Could you check a few things on this model? Use its own coordinates, in mm. A direction names the side the tool comes from. Coordinates: 2 decimals unless noted, no trailing zeros. Order: outer loops, then holes, each group sorted by start corner. A loop starts at its lowest first (then second) coordinate and runs counter-clockwise, first axis right, second up.
```python
from build123d import *

# Parameters (mm, degrees)
F0_R     = 20.955
F1_DEPTH = 6.35
F3_R     = 13.97
F4_DEPTH = 38.1
F5_R     = 7.62
F2_R     = 1.905
F7_DEPTH = 2.54
F6_R     = 1.905
F8_DEPTH = 2.54


with BuildPart() as f1:
    # F0 (on Top) → F1 (new body)
    with BuildSketch(Plane.XY):
        Circle(F0_R)
    extrude(amount=F1_DEPTH)

    # F3 (on face) → F4 (join)
    with BuildSketch(Plane(origin=(0, 0, 0), x_dir=(1, 0, 0), z_dir=(0, 0, -1))):
        Circle(F3_R)
    extrude(amount=F4_DEPTH)

    # F5
    f5_edges = [f1.edges().sort_by_distance(p)[0] for p in [
        (-13.97, 0, -38.1),
    ]]
    fillet(f5_edges, radius=F5_R)

    # F2 (on face) → F7 (cut)
    with BuildSketch(Plane.XY.offset(6.35)):
        with Locations((10.57046, -10.57046)):
            Circle(F2_R)
    extrude(amount=-F7_DEPTH, mode=Mode.SUBTRACT)

    # F6 (on face) → F8 (cut)
    with BuildSketch(Plane.XY.offset(6.35)):
        with Locations((-10.57046, -10.57046)):
            Circle(F6_R)
        with Locations((10.57046, 10.57046)):
            Circle(F6_R)
        with Locations((-10.57046, 10.57046)):
            Circle(F6_R)
        Circle(F6_R)
        with Locations((0, 14.948888)):
            Circle(F6_R)
        with Locations((14.948888, 0)):
            Circle(F6_R)
        with Locations((0, -14.948888)):
            Circle(F6_R)
        with Locations((10.57046, -10.57046)):
            Circle(F6_R)
        with Locations((-14.948888, 0)):
            Circle(F6_R)
    extrude(amount=-F8_DEPTH, mode=Mode.SUBTRACT)


solid = f1.part
```
Item 1: Which directions (+Z, -Z, +X, -X, +Y, -Y) give clear straight access to the entire face, cutting with the end or side of a thin tool? Please do faces 1 (the face through (-2.728, 20.777, 3.131)), 2 (the face through (4, -14, 0)), 3 (the face through (12.39, -10, 5.1)).
Item 2: Suppose I cut it at A-A (x = 15). List the corners of the cut face in (y, z) for me, and give its area (3 significant figures).
Item 3: Thinking about a two-plate mould opening in X: for faces 4 (the face through (0, 0, -38.1)), 5 (the face through (-1.82, -13.85, -15.03)), 6 (the face through (12.4, 11.1, 5.1)), which applies, +X half, -X half, draft (parallel to the pull), parting line (faces both ways), or undercut?
Item 4: Suppose I cut it at C-C (x = -16). List the corners of the cut face in (y, z) for me.
Item 5: Suppose I cut it at B-B (z = -27.5). List the corners of the cut face in (x, y) for me.
Item 6: Suppose I cut it at D-D (y = 18.5). List the corners of the cut face in (x, z) for me, and give its area (3 significant figures).
Item 7: I need wall thicknesses on line 1 (Y direction, x = 0, z = 5.1) (3 decimals); line 2 (Z direction, x = 10, y = 14.5); line 3 (Y direction, x = 0, z = -10). Which ranges of each line are inside material? Lowest first, please.
Item 8: For pin 1 Ø3 at (x, y) = (-10.5, -10.5) entering from +Z; pin 2 Ø1 at (y, z) = (-2.5, -15) entering from +X; pin 3 Ø2 at (y, z) = (9.5, -27) entering from +X; pin 4 Ø2 at (x, z) = (16, -7) entering from +Y, each with a flat end and sliding along its axis, tell me the tip position at first contact or that it passes through.
Geometry results:
1. face 1: +Z, -Z
1. face 2: -Z
1. face 3: +Z
2. outline: (-14.63, 0) - (14.63, 0) - (14.63, 6.35) - (1.9, 6.35) - (1.9, 3.81) - (-1.9, 3.81) - (-1.9, 6.35) - (-14.63, 6.35) - close
2. area: 176 mm2
3. face 4: draft
3. face 5: parting line
3. face 6: undercut
4. outline: (-13.53, 0) - (13.53, 0) - (13.53, 6.35) - (1.59, 6.35) - (1.59, 3.81) - (-1.59, 3.81) - (-1.59, 6.35) - (-13.53, 6.35) - close
5. outline: circle Ø27.94 at (0, 0)
6. outline: (-9.84, 0) - (9.84, 0) - (9.84, 6.35) - (-9.84, 6.35) - close
6. area: 125 mm2
7. line 1: y = -20.955 to -16.854, -13.044 to -1.905, 1.905 to 13.044, 16.854 to 20.955
7. line 2: z = 0 to 6.35
7. line 3: y = -13.97 to 13.97
8. pin 1: stops at z = 3.81
8. pin 2: stops at x = 13.83
8. pin 3: stops at x = 11.09
8. pin 4: passes through
